Geometry: final body of the model. Coordinates: model frame, mm. A direction names the side the tool comes from. Coordinates: 2 decimals unless noted, no trailing zeros. Write each loop counter-clockwise with the first axis right and the second up, starting at its lowest first coordinate (ties: lowest second). Pieces come first, ordered by that corner, then holes. Notation, with made-up numbers: (7.5, 12.5) -> (54.5, 12.5) arc R28 ccw to (54.5, 38.5) -> close; hole circle Ø8 at (52.25, 57). An arc over 180 degrees is marked (long way). One line per item, written item: value.
Autodesk Fusion 360 part; units mm, degrees
sketch "Sketch1" plane through (0, 0, 0) normal (0, 1, 0) x (1, 0, 0)
  line L0 (1.75, 0) -> (22.5, 0)
  arc A0 (-33.6984, -4) -> (-33.6984, 4) centre (-18, 0) ccw
  arc A1 (-31.6635, -1) -> (-31.6635, 1) centre (-18, 0) ccw
  line L1 (-33.6984, 4) -> (-40.6984, 4)
  line L2 (-40.6984, 4) -> (-40.6984, 1)
  line L3 (-40.6984, 1) -> (-31.6635, 1)
  line L4 (-33.6984, -4) -> (-40.6984, -4)
  line L5 (-40.6984, -4) -> (-40.6984, -1)
  line L6 (-40.6984, -1) -> (-31.6635, -1)
  line L7 (-18, 0) -> (-40.6984, 0) construction
  circle A2 centre (-18, 0) radius 12.9205 construction
  line L8 (0, -16.2) -> (0, 16.2)
  line L9 (0, 16.2) -> (-18, 16.2)
  line L10 (0, -16.2) -> (-18, -16.2)
  line L11 (0, 16.2) -> (18, 16.2)
  line L12 (33.6984, -4) -> (40.6984, -4)
  arc A3 (31.6635, 1) -> (31.6635, -1) centre (18, 0) ccw
  circle A4 centre (18, 0) radius 12.9205 construction
  line L13 (40.6984, -4) -> (40.6984, -1)
  line L14 (40.6984, -1) -> (31.6635, -1)
  line L15 (40.6984, 4) -> (40.6984, 1)
  line L16 (18, 0) -> (40.6984, 0) construction
  line L17 (40.6984, 1) -> (31.6635, 1)
  line L18 (0, -16.2) -> (18, -16.2)
  line L19 (33.6984, 4) -> (40.6984, 4)
  line L20 (0, -16.2) -> (0, 16.2)
  arc A5 (33.6984, 4) -> (33.6984, -4) centre (18, 0) ccw
  point P0 (-1.75, 0)
  dimension "d2" = 18
  dimension "d16" = 7
  dimension "d17" = 3
  dimension "d18" = 7
  dimension "d19" = 3
  dimension "d20" = 25.841
  dimension "d21" = 32.4
  dimension "d22" = 13.7
  dimension "d23" = 16.2
extrude "Extrude1" add sketch "Sketch1" along normal blind 7
hole "Hole1" at (-37.1984, 3.5, -4) direction (0, 0, 1) diameter 3.2 depth 8 tip angle 180
hole "Hole2" at (37.1984, 3.5, 4) direction (0, 0, -1) diameter 3.2 depth 8 tip angle 180
sketch "Sketch3" plane through (0, 0, 16.2) normal (0, 0, 1) x (1, 0, 0)
  line L0 (-18, 0) -> (18, 0)
  line L1 (18, 0) -> (18, 7)
  line L2 (18, 7) -> (-18, 7)
  line L3 (-18, 7) -> (-18, 0)
  line L4 (0, 0) -> (0, 7) construction
  line L5 (-2, 7) -> (-6, 7)
  line L6 (-6, 7) -> (-6, 0)
  line L7 (-6, 0) -> (-2, 0)
  line L8 (-2, 0) -> (-2, 7)
  line L9 (2, 7) -> (6, 7)
  line L10 (6, 7) -> (6, 0)
  line L11 (6, 0) -> (2, 0)
  line L12 (2, 0) -> (2, 7)
  dimension "d35" = 4
  dimension "d36" = 7
  dimension "d37" = 2
  dimension "d38" = 4
  dimension "d39" = 7
  dimension "d40" = 2
sketch "Sketch4" plane through (0, 0, -16.2) normal (0, 0, -1) x (-1, 0, 0)
  line L0 (-18, 0) -> (18, 0)
  line L1 (18, 0) -> (18, 7)
  line L2 (18, 7) -> (-18, 7)
  line L3 (-18, 7) -> (-18, 0)
  line L4 (0, 0) -> (0, 7) construction
  line L5 (-6, 7) -> (-2, 7)
  line L6 (-2, 7) -> (-2, 0)
  line L7 (-2, 0) -> (-6, 0)
  line L8 (-6, 0) -> (-6, 7)
  line L9 (2, 7) -> (6, 7)
  line L10 (6, 7) -> (6, 0)
  line L11 (6, 0) -> (2, 0)
  line L12 (2, 0) -> (2, 7)
  dimension "d41" = 2
  dimension "d42" = 2
  dimension "d43" = 4
  dimension "d44" = 4
extrude "Extrude2" add sketch "Sketch4" along normal blind 15 contours L0 L2 L5 L6 L7 L8 | L0 L2 L9 L10 L11 L12
extrude "Extrude3" add sketch "Sketch3" along normal blind 15 contours L0 L2 L5 L6 L7 L8 | L0 L2 L9 L10 L11 L12
hole "Hole3" at (-6, 3.5, -27.7) direction (1, 0, 0) diameter 3.1 depth 12 tip angle 180
hole "Hole4" at (-6, 3.5, -19.7) direction (1, 0, 0) diameter 3.1 depth 12 tip angle 180
hole "Hole5" at (6, 3.5, 27.7) direction (-1, 0, 0) diameter 3.1 depth 12 tip angle 180
hole "Hole6" at (6, 3.5, 19.7) direction (-1, 0, 0) diameter 3.1 depth 12 tip angle 180
(1) First-contact query: pin 1 (3.5 mm diameter, centred on y = 3.5, z = -19.7, fed in from -X); pin 2 (4 mm diameter, centred on x = -37.2, y = 3.5, fed in from -Z); pin 3 (3.5 mm diameter, centred on x = -13, y = 4, fed in from +Z); pin 4 (3 mm diameter, centred on x = 37.2, y = 3.5, fed in from +Z). Flat tips, straight axial feed; report the tip coordinate or a pass-through.
Responses:
pin 1: stops at x = -6
pin 2: stops at z = -4
pin 3: stops at z = 16.2
pin 4: passes through
(2) Section C-C (x = -20.5). Return the cut outline in (y, z).
Responses:
outline: (0, -16.01) -> (7, -16.01) -> (7, -13.47) -> (0, -13.47) -> close; (0, 13.47) -> (7, 13.47) -> (7, 16.01) -> (0, 16.01) -> close
(3) Pull-direction query (Y, two-part tool) for faces 1 (the cylindrical face through (-35.636, 3.153, -2.479)), 2 (the flat face through (0, 0, 0)), 3 (the flat face through (6, 3, -24)), 4 (the cylindrical face through (-4.03, 3.43, 29.25)); classes: released by +Y, released by -Y, zero draft, split by the parting line, or undercut.
Responses:
face 1: undercut
face 2: released by -Y
face 3: zero draft
face 4: undercut
(4) Section B-B (z = -2.5). Return the cut outline in (x, y).
Responses:
outline: (-40.7, 0) -> (-31.47, 0) -> (-31.47, 7) -> (-40.7, 7) -> close; (-4.53, 0) -> (4.53, 0) -> (4.53, 7) -> (-4.53, 7) -> close; (31.47, 0) -> (40.7, 0) -> (40.7, 7) -> (31.47, 7) -> close; hole circle Ø3.2 at (-37.2, 3.5); hole circle Ø3.2 at (37.2, 3.5)
(5) Line query: line 1 (Z direction, x = -3.7, y = 3.5); line 2 (Z direction, x = 34, y = 4.75); line 3 (X direction, y = 4.5, z = 5.5). Output: solid intervals per line, ascending. Write a range as [from, to].
Responses:
line 1: z = [-31.2, -29.25], [-26.15, -21.25], [-18.15, 18.15], [21.25, 26.15], [29.25, 31.2]
line 2: z = [-4, -1], [1, 4]
line 3: x = [-33.24, -30.55], [-5.45, 5.45], [30.55, 33.24]
(6) Section D-D (y = 3.5). State how many separate pieces and enclosed holes the cut face has, then the cut area to 3 significant figures.
Responses:
separate pieces: 13
enclosed holes: 0
area: 985 mm2
(7) Section A-A (z = 24). Return the cut outline in (x, y).
Responses:
outline: (-6, 0) -> (-2, 0) -> (-2, 7) -> (-6, 7) -> close; (2, 0) -> (6, 0) -> (6, 7) -> (2, 7) -> close
(8) Reachability of faces 5 (the flat face through (12, 3, 16.2)), 6 (the flat face through (2, 4, -24)), 7 (the flat face through (-35.6, 2.7, -4)), 8 (the flat face through (35, 3, -1)), 9 (the flat face through (-35, 3, 1)) from +Z, -Z, +X, -X, +Y, -Y: full face, straight path, thin tool, end or side. Return the list, or none.
Responses:
face 5: +Z, +X, +Y, -Y
face 6: -Z, +Y, -Y
face 7: -Z, -X, +Y, -Y
face 8: +X, +Y, -Y
face 9: -X, +Y, -Y
